The listing builds one solid part. Answer for the finished solid, in the listing's coordinates (mm). A direction names the side the tool comes from. Coordinates: 2 decimals unless noted, no trailing zeros. Order: outer loops, then holes, each group sorted by start corner. A loop starts at its lowest first (then second) coordinate and runs counter-clockwise, first axis right, second up.
Solid Edge part; units mm, degrees
sketch "Sketch1" plane through (0, 0, 0) normal (0, 0, 1) x (1, 0, 0)
  line L0 (-175, -175) -> (175, -175)
  line L1 (175, -175) -> (175, 175)
  line L2 (175, 175) -> (-175, 175)
  line L3 (-175, 175) -> (-175, -175)
  dimension "D1" = 175
  dimension "D2" = 175
extrude "Protrusion1" add sketch "Sketch1" along normal blind 7.5
sketch "Sketch2" plane through (0, 0, 7.5) normal (0, 0, 1) x (1, 0, 0)
  circle A0 centre (0, 0) radius 75
  circle A1 centre (0, 0) radius 60
extrude "Wyciągnięcie_2" add sketch "Sketch2" along normal blind 100
sketch "Sketch3" plane through (0, 0, 107.5) normal (0, 0, 1) x (0, 1, 0)
  circle A0 centre (0, 0) radius 82.5
  circle A1 centre (0, 0) radius 75
extrude "Wyciągnięcie_3" add sketch "Sketch3" against normal blind 5
sketch "Sketch4" plane through (0, 0, 77.2) normal (0, 0, 1) x (1, 0, 0)
  line L0 (-64.2773, 24.6751) -> (30.7757, -61.5897)
  line L1 (-39.7647, 56.2067) -> (61.855, -30.2388)
  arc A0 (-64.2773, 24.6751) -> (-39.7647, 56.2067) centre (0, 0) cw
  line L2 (30.7757, -61.5897) -> (61.855, -30.2388)
extrude "Wyciągnięcie_4" add sketch "Sketch4" against normal blind 3.5
hole "Otwór_1" at (-67.6252, 2.2673, 0) direction (0, 0, 1) diameter 2.459 depth 10.5
sketch "Sketch5" plane through (0, 0, 0) normal (0, 0, -1) x (1, 0, 0)
  circle A0 centre (-67.6252, -2.2673) radius 2.75
extrude "Wycięcie_1" cut sketch "Sketch5" against normal blind 2.5
pattern_circular "Pattern1" count 4 over 360 about axis through (0, 0, 0) along (0, 0, 1) of "Wycięcie_1", "Otwór_1"
(1) The mould has two halves that part along Z. Classify faces 3 (the face through (-59.94, -2.64, 56.8)), 4 (the face through (-2, 2, 0)), 5 (the face through (-9.764, -74.362, 54.335)), 6 (the face through (6, -61, 107.5)): released by +Z, released by -Z, zero draft, split by the parting line, or undercut.
(2) Find section A-A (y = -19). Write down the section's boundary in (x, z), and give its area (3 significant figures).
(3) Consider line 1 (Z direction, x = -39, y = 14.5); line 2 (Y direction, x = 21, z = 75.5); line 3 (Z direction, x = -91, y = -89). Determine where each line is inside the solid, lowest interval first.
(4) Find section B-B (z = 60.5). Write down the section's boundary in (x, y), and give its area (3 significant figures).
(5) Find section D-D (x = 135). Write down the section's boundary in (y, z).
(6) Find section C-C (y = 35). Write down the section's boundary in (x, z).
(7) For faces 1 (the face through (18, -73, 102.5)), 2 (the face through (80.54, -17.88, 105.04)), determine the directions among +Z, -Z, +X, -X, +Y, -Y from which every point of the face is accessible in a straight line to the end or side of a thin tool.
(8) Each of these flat-tipped pins is pushed along its axis until it touches: pin 1 Ø8 at (x, z) = (37.5, 25.5) entering from -Y; pin 2 Ø5 at (x, y) = (-2.27, -67.63) entering from -Z; pin 3 Ø1 at (y, z) = (8, 52) entering from -X; pin 4 Ø4 at (x, z) = (-78.5, 81.5) entering from +Y. Where does it stop, or does it pass through?
Findings below:
1. face 3: undercut
1. face 4: released by -Z
1. face 5: undercut
1. face 6: released by +Z
2. outline: (-175, 0) - (175, 0) - (175, 7.5) - (72.55, 7.5) - (72.55, 102.5) - (80.28, 102.5) - (80.28, 107.5) - (56.91, 107.5) - (56.91, 7.5) - (-56.91, 7.5) - (-56.91, 107.5) - (-80.28, 107.5) - (-80.28, 102.5) - (-72.55, 102.5) - (-72.55, 7.5) - (-175, 7.5) - close; (-16.15, 73.7) - (48.64, 73.7) - (48.64, 77.2) - (-16.15, 77.2) - close
2. area: 6,060 mm2
3. line 1: z = 0 to 7.5, 73.7 to 77.2
3. line 2: y = -72 to -56.2, -52.72 to 4.52, 56.2 to 72
3. line 3: z = 0 to 7.5
4. outline: circle Ø150 at (0, 0); hole circle Ø120 at (0, 0)
4. area: 6,360 mm2
5. outline: (-175, 0) - (175, 0) - (175, 7.5) - (-175, 7.5) - close
6. outline: (-175, 0) - (175, 0) - (175, 7.5) - (66.33, 7.5) - (66.33, 102.5) - (74.71, 102.5) - (74.71, 107.5) - (48.73, 107.5) - (48.73, 7.5) - (-48.73, 7.5) - (-48.73, 73.7) - (-14.84, 73.7) - (-14.84, 77.2) - (-48.73, 77.2) - (-48.73, 107.5) - (-74.71, 107.5) - (-74.71, 102.5) - (-66.33, 102.5) - (-66.33, 7.5) - (-175, 7.5) - close
7. face 1: none
7. face 2: +Z
8. pin 1: stops at y = -67.1
8. pin 2: stops at z = 2.5
8. pin 3: stops at x = -74.62
8. pin 4: passes through
